Input: part model. Units: mm. Frame: model coordinates. A direction names the side the tool comes from. Give positions to 0.01 mm unless a question says otherwise; leave off trailing zeros. Loops run counter-clockwise (first coordinate to the right, second up) from the corner with the lowest first, then second, coordinate; pieces in that order, holes last. Notation, with made-up numbers: M 30,84.5 L 35,84.5 A36 cw 35,122.5 Z; hole C -19.75,12 d5. An arc over 180 degrees is marked long. Answer as a JSON object with one key per item and string values. Group by question number.
1) Section query A-A on y = 0.5. Return loops of the section in (x, z) (3 decimals).
2) Section query D-D on y = 86.5. Return loops of the section in (x, z) (3 decimals), plus the area to 3 significant figures.
3) Ray query, L1, parallel to X at y = 7, z = 2.4; L2, parallel to Y at x = -75, z = 2. Return the intervals inside material, ascending.
4) Access query for faces 1 (the flat face through (-29.18, 28.86, 1.57)), 2 (the flat face through (-84.6, 85.11, 1.57)). Directions: +Z, -Z, +X, -X, +Y, -Y. A direction counts if a zero-diameter tool reaches every point of the face in a straight line with its end or side. Return the directions, or none.
5) Section query B-B on x = -99. Return loops of the section in (y, z) (3 decimals).
6) Section query C-C on z = 1.7. Count the separate pieces of the cut face and the enclosed holes in it, plus the area to 3 significant figures.
7) Draft query along Y for faces 3 (the flat face through (-85.11, -84.6, 1.57)), 4 (the flat face through (85.11, 84.6, 1.57)), 5 (the cylindrical face through (-106.096, -43.619, 1.565)). Return one class per face: +Y half, -Y half, draft (parallel to the pull), parting line (faces both ways), or undercut.
from build123d import *

# Parameters (mm, degrees)
SKETCH1_R           = 2.5
SKETCH1_R_2         = 1.5
BOSS_EXTRUDE2_DEPTH = 3.175
FILLET2_R           = 2


with BuildPart() as part:
    # Sketch1 → Boss-Extrude2 (new body)
    with BuildSketch(Plane.XY):
        with BuildLine():
            Line((-120, 26.433190344), (-120, -26.433190344))
            ThreePointArc((-120, -26.433190344), (-105.978758658, -43.899668257), (-103.544901199, -66.165098801))
            Line((-103.544901199, -66.165098801), (-66.165098801, -103.544901199))
            ThreePointArc((-66.165098801, -103.544901199), (-43.899668257, -105.978758658), (-26.433190344, -120))
            Line((-26.433190344, -120), (26.433190344, -120))
            ThreePointArc((26.433190344, -120), (43.899668257, -105.978758658), (66.165098801, -103.544901199))
            Line((66.165098801, -103.544901199), (103.544901199, -66.165098801))
            ThreePointArc((103.544901199, -66.165098801), (105.978758658, -43.899668257), (120, -26.433190344))
            Line((120, -26.433190344), (120, 26.433190344))
            ThreePointArc((120, 26.433190344), (105.978758658, 43.899668257), (103.544901199, 66.165098801))
            Line((103.544901199, 66.165098801), (66.165098801, 103.544901199))
            ThreePointArc((66.165098801, 103.544901199), (43.899668257, 105.978758658), (26.433190344, 120))
            Line((26.433190344, 120), (-26.433190344, 120))
            ThreePointArc((-26.433190344, 120), (-43.899668257, 105.978758658), (-66.165098801, 103.544901199))
            Line((-66.165098801, 103.544901199), (-103.544901199, 66.165098801))
            ThreePointArc((-103.544901199, 66.165098801), (-105.978758658, 43.899668257), (-120, 26.433190344))
        make_face()
        with Locations((-91.926067812, 70.712864376)):
            Circle(SKETCH1_R, mode=Mode.SUBTRACT)
        with Locations((-70.712864376, 91.926067812)):
            Circle(SKETCH1_R, mode=Mode.SUBTRACT)
        with Locations((-25.485281374, 46.69848481)):
            Circle(SKETCH1_R, mode=Mode.SUBTRACT)
        with Locations((-46.69848481, 25.485281374)):
            Circle(SKETCH1_R, mode=Mode.SUBTRACT)
        with Locations((-15, 115)):
            Circle(SKETCH1_R, mode=Mode.SUBTRACT)
        with Locations((-15, 51.04163056)):
            Circle(SKETCH1_R, mode=Mode.SUBTRACT)
        with Locations((-115, 15)):
            Circle(SKETCH1_R, mode=Mode.SUBTRACT)
        with Locations((-51.04163056, 15)):
            Circle(SKETCH1_R, mode=Mode.SUBTRACT)
        with Locations((-75, 60)):
            Circle(SKETCH1_R_2, mode=Mode.SUBTRACT)
        with Locations((-50, 60)):
            Circle(SKETCH1_R_2, mode=Mode.SUBTRACT)
        with Locations((-43.162950904, 43.162950904)):
            Circle(SKETCH1_R_2, mode=Mode.SUBTRACT)
        with Locations((0, 61.04163056)):
            Circle(SKETCH1_R_2, mode=Mode.SUBTRACT)
        with Locations((-75, 26.433190344)):
            Circle(SKETCH1_R_2, mode=Mode.SUBTRACT)
        with Locations(Location((75, 26.433190344, 0), (0, 0, 180))):
            Circle(SKETCH1_R_2, mode=Mode.SUBTRACT)
        with Locations(Location((43.162950904, 43.162950904, 0), (0, 0, 180))):
            Circle(SKETCH1_R_2, mode=Mode.SUBTRACT)
        with Locations(Location((50, 60, 0), (0, 0, 180))):
            Circle(SKETCH1_R_2, mode=Mode.SUBTRACT)
        with Locations(Location((75, 60, 0), (0, 0, 180))):
            Circle(SKETCH1_R_2, mode=Mode.SUBTRACT)
        with Locations(Location((51.04163056, 15, 0), (0, 0, 180))):
            Circle(SKETCH1_R, mode=Mode.SUBTRACT)
        with Locations(Location((115, 15, 0), (0, 0, 180))):
            Circle(SKETCH1_R, mode=Mode.SUBTRACT)
        with Locations(Location((15, 51.04163056, 0), (0, 0, 180))):
            Circle(SKETCH1_R, mode=Mode.SUBTRACT)
        with Locations(Location((15, 115, 0), (0, 0, 180))):
            Circle(SKETCH1_R, mode=Mode.SUBTRACT)
        with Locations(Location((46.69848481, 25.485281374, 0), (0, 0, 180))):
            Circle(SKETCH1_R, mode=Mode.SUBTRACT)
        with Locations(Location((25.485281374, 46.69848481, 0), (0, 0, 180))):
            Circle(SKETCH1_R, mode=Mode.SUBTRACT)
        with Locations(Location((70.712864376, 91.926067812, 0), (0, 0, 180))):
            Circle(SKETCH1_R, mode=Mode.SUBTRACT)
        with Locations(Location((91.926067812, 70.712864376, 0), (0, 0, 180))):
            Circle(SKETCH1_R, mode=Mode.SUBTRACT)
        with Locations((91.926067812, -70.712864376)):
            Circle(SKETCH1_R, mode=Mode.SUBTRACT)
        with Locations((70.712864376, -91.926067812)):
            Circle(SKETCH1_R, mode=Mode.SUBTRACT)
        with Locations((25.485281374, -46.69848481)):
            Circle(SKETCH1_R, mode=Mode.SUBTRACT)
        with Locations((46.69848481, -25.485281374)):
            Circle(SKETCH1_R, mode=Mode.SUBTRACT)
        with Locations((15, -115)):
            Circle(SKETCH1_R, mode=Mode.SUBTRACT)
        with Locations((15, -51.04163056)):
            Circle(SKETCH1_R, mode=Mode.SUBTRACT)
        with Locations((115, -15)):
            Circle(SKETCH1_R, mode=Mode.SUBTRACT)
        with Locations((51.04163056, -15)):
            Circle(SKETCH1_R, mode=Mode.SUBTRACT)
        with Locations((75, -60)):
            Circle(SKETCH1_R_2, mode=Mode.SUBTRACT)
        with Locations((50, -60)):
            Circle(SKETCH1_R_2, mode=Mode.SUBTRACT)
        with Locations((43.162950904, -43.162950904)):
            Circle(SKETCH1_R_2, mode=Mode.SUBTRACT)
        with Locations((75, -26.433190344)):
            Circle(SKETCH1_R_2, mode=Mode.SUBTRACT)
        with Locations(Location((-75, -26.433190344, 0), (0, 0, 180))):
            Circle(SKETCH1_R_2, mode=Mode.SUBTRACT)
        with Locations(Location((0, -61.04163056, 0), (0, 0, 180))):
            Circle(SKETCH1_R_2, mode=Mode.SUBTRACT)
        with Locations(Location((-43.162950904, -43.162950904, 0), (0, 0, 180))):
            Circle(SKETCH1_R_2, mode=Mode.SUBTRACT)
        with Locations(Location((-50, -60, 0), (0, 0, 180))):
            Circle(SKETCH1_R_2, mode=Mode.SUBTRACT)
        with Locations(Location((-75, -60, 0), (0, 0, 180))):
            Circle(SKETCH1_R_2, mode=Mode.SUBTRACT)
        with Locations(Location((-51.04163056, -15, 0), (0, 0, 180))):
            Circle(SKETCH1_R, mode=Mode.SUBTRACT)
        with Locations(Location((-115, -15, 0), (0, 0, 180))):
            Circle(SKETCH1_R, mode=Mode.SUBTRACT)
        with Locations(Location((-15, -51.04163056, 0), (0, 0, 180))):
            Circle(SKETCH1_R, mode=Mode.SUBTRACT)
        with Locations(Location((-15, -115, 0), (0, 0, 180))):
            Circle(SKETCH1_R, mode=Mode.SUBTRACT)
        with Locations(Location((-46.69848481, -25.485281374, 0), (0, 0, 180))):
            Circle(SKETCH1_R, mode=Mode.SUBTRACT)
        with Locations(Location((-25.485281374, -46.69848481, 0), (0, 0, 180))):
            Circle(SKETCH1_R, mode=Mode.SUBTRACT)
        with Locations(Location((-70.712864376, -91.926067812, 0), (0, 0, 180))):
            Circle(SKETCH1_R, mode=Mode.SUBTRACT)
        with Locations(Location((-91.926067812, -70.712864376, 0), (0, 0, 180))):
            Circle(SKETCH1_R, mode=Mode.SUBTRACT)
        with Locations((-80, 15.849242405)):
            Circle(SKETCH1_R, mode=Mode.SUBTRACT)
        with Locations((-80, -15.849242405)):
            Circle(SKETCH1_R, mode=Mode.SUBTRACT)
        with Locations((80, -15)):
            Circle(SKETCH1_R, mode=Mode.SUBTRACT)
        with Locations((80, 15)):
            Circle(SKETCH1_R, mode=Mode.SUBTRACT)
        Polygon((-41.04163056, 17), (-17, 41.04163056), (17, 41.04163056), (41.04163056, 17), (41.04163056, -17), (17, -41.04163056), (-17, -41.04163056), (-41.04163056, -17), align=None, mode=Mode.SUBTRACT)
    extrude(amount=BOSS_EXTRUDE2_DEPTH)

    # Fillet2
    fillet2_edges = [part.edges().sort_by_distance(p)[0] for p in [
        (-26.433190344, 120, 1.5875),
        (26.433190344, 120, 1.5875),
        (66.165098801, 103.544901199, 1.5875),
        (103.544901199, 66.165098801, 1.5875),
        (120, 26.433190344, 1.5875),
        (120, -26.433190344, 1.5875),
        (103.544901199, -66.165098801, 1.5875),
        (66.165098801, -103.544901199, 1.5875),
        (26.433190344, -120, 1.5875),
        (-26.433190344, -120, 1.5875),
        (-66.165098801, -103.544901199, 1.5875),
        (-103.544901199, -66.165098801, 1.5875),
        (-120, -26.433190344, 1.5875),
        (-120, 26.433190344, 1.5875),
        (-103.544901199, 66.165098801, 1.5875),
        (-66.165098801, 103.544901199, 1.5875),
        (-41.04163056, 17, 1.5875),
        (-41.04163056, -17, 1.5875),
        (-17, -41.04163056, 1.5875),
        (17, -41.04163056, 1.5875),
        (41.04163056, -17, 1.5875),
        (41.04163056, 17, 1.5875),
        (17, 41.04163056, 1.5875),
        (-17, 41.04163056, 1.5875),
    ]]
    fillet(fillet2_edges, radius=FILLET2_R)


solid = part.part
Output:
{
 "1": {"outline": "M -120,0 L -41.042,0 L -41.042,3.175 L -120,3.175 Z; M 41.042,0 L 120,0 L 120,3.175 L 41.042,3.175 Z"},
 "2": {"outline": "M -83.21,0 L 83.21,0 L 83.21,3.175 L -83.21,3.175 Z", "area": "528 mm^2"},
 "3": {"L1": "x = -120 to -41.04, 41.04 to 120", "L2": "y = -94.71 to -61.5, -58.5 to -27.93, -24.93 to 24.93, 27.93 to 58.5, 61.5 to 94.71"},
 "4": {"face 1": "+Z, -Z", "face 2": "+Z, -Z, -X, +Y"},
 "5": {"outline": "M -70.71,0 L 70.71,0 L 70.71,3.175 L -70.71,3.175 Z"},
 "6": {"separate pieces": "1", "enclosed holes": "55", "area": "38,300 mm^2"},
 "7": {"face 3": "-Y half", "face 4": "+Y half", "face 5": "undercut"}
}
